```python
from build123d import *

# Parameters (mm, degrees)
SKETCH1_R               = 17
BOSS_EXTRUDE1_DEPTH     = 4.4
CAVITY1_OUTLINE_R       = 3.15
CAVITY1_DEPTH           = 3.283595969
CAVITY1_START           = 1.183595969
CAVITY1_2_OUTLINE_R     = 3.15
CAVITY1_2_OUTLINE_R_2   = 1.575
CAVITY1_2_DEPTH         = 2.1
SKETCH9_R               = 12.8
BOSS_EXTRUDE3_DEPTH     = 5.6
BOSS_EXTRUDE8_DEPTH     = 8
SKETCH2_R               = 0.6
CUT_EXTRUDE1_DEPTH      = 31.033314835
CIRPATTERN1_COUNT       = 6
CUT_EXTRUDE3_DEPTH      = 31.033314835
CUT_EXTRUDE3_DEPTH_BACK = 4
SKETCH4_R               = 4
SKETCH6_R               = 1.8
CUT_EXTRUDE4_DEPTH      = 31.033314835
FILLET1_START           = 10
FILLET1_DEPTH           = 9
CUT_EXTRUDE5_DEPTH      = 27.038433133
CUT_EXTRUDE5_DEPTH_BACK = 5.6


with BuildPart() as part:
    # Sketch1 → Boss-Extrude1 (new body)
    with BuildSketch(Plane.XY):
        Circle(SKETCH1_R)
    extrude(amount=BOSS_EXTRUDE1_DEPTH)

    # Cavity1: read off the stored shape, not the designer's step
    # Cavity1 outline → Cavity1 (cut)
    with BuildSketch(Plane.XY):
        with BuildLine():
            Line((3.9375, 6.819950055), (2.048148228, 15.163776711))
            ThreePointArc((2.048148228, 15.163776711), (0, 16.8), (-2.048148228, 15.163776711))
            Line((-2.048148228, 15.163776711), (-3.9375, 6.819950055))
            Line((-3.9375, 6.819950055), (-12.108141735, 9.355636751))
            ThreePointArc((-12.108141735, 9.355636751), (-14.549226784, 8.4), (-14.156289963, 5.80813996))
            Line((-14.156289963, 5.80813996), (-7.875, 0))
            Line((-7.875, 0), (-14.156289963, -5.80813996))
            ThreePointArc((-14.156289963, -5.80813996), (-14.549226784, -8.4), (-12.108141735, -9.355636751))
            Line((-12.108141735, -9.355636751), (-3.9375, -6.819950055))
            Line((-3.9375, -6.819950055), (-2.048148228, -15.163776711))
            ThreePointArc((-2.048148228, -15.163776711), (0, -16.8), (2.048148228, -15.163776711))
            Line((2.048148228, -15.163776711), (3.9375, -6.819950055))
            Line((3.9375, -6.819950055), (12.108141735, -9.355636751))
            ThreePointArc((12.108141735, -9.355636751), (14.549226784, -8.4), (14.156289963, -5.80813996))
            Line((14.156289963, -5.80813996), (7.875, 0))
            Line((7.875, 0), (14.156289963, 5.80813996))
            ThreePointArc((14.156289963, 5.80813996), (14.549226784, 8.4), (12.108141735, 9.355636751))
            Line((12.108141735, 9.355636751), (3.9375, 6.819950055))
        make_face()
        Circle(CAVITY1_OUTLINE_R, mode=Mode.SUBTRACT)
    extrude(amount=CAVITY1_DEPTH, mode=Mode.SUBTRACT)

    # Cavity1 2 outline → Cavity1 2 (cut)
    with BuildSketch(Plane.XY.offset(CAVITY1_START)):
        Circle(CAVITY1_2_OUTLINE_R)
        Circle(CAVITY1_2_OUTLINE_R_2, mode=Mode.SUBTRACT)
    extrude(amount=CAVITY1_2_DEPTH, mode=Mode.SUBTRACT)

    # Sketch9 → Boss-Extrude3 (add)
    with BuildSketch(Plane.XY.offset(4.4)):
        Circle(SKETCH9_R)
    extrude(amount=BOSS_EXTRUDE3_DEPTH)

    # Sketch12 → Boss-Extrude8 (add)
    with BuildSketch(Plane.XY.offset(10)):
        Polygon((3.9, -6.75499815), (7.8, 0), (3.9, 6.75499815), (-3.9, 6.75499815), (-7.8, 0), (-3.9, -6.75499815), align=None)
    extrude(amount=BOSS_EXTRUDE8_DEPTH)

    # Sketch2 → Cut-Extrude1 (cut, through all)
    with BuildSketch(Plane(origin=(0, 0, 0), x_dir=(-1, 0, 0), z_dir=(0, 0, -1))):
        with Locations(Location((0, 13.5, 0), (0, 0, 180))):
            Circle(SKETCH2_R)
        with Locations(Location((0, 10.5, 0), (0, 0, 180))):
            Circle(SKETCH2_R)
        with Locations(Location((0, 7.5, 0), (0, 0, 180))):
            Circle(SKETCH2_R)
    cut_extrude1 = extrude(amount=-CUT_EXTRUDE1_DEPTH, mode=Mode.SUBTRACT)

    # CirPattern1: Cut-Extrude1 ×6 about axis
    cirpattern1_axis = Axis((0, 0, 0), (0, 0, 1))
    for i in range(1, CIRPATTERN1_COUNT):
        add(cut_extrude1.rotate(cirpattern1_axis, i * 360 / CIRPATTERN1_COUNT), mode=Mode.SUBTRACT)

    # Sketch4 → Cut-Extrude3 (cut, two sides: drawn at the far end of the back side and taken through both)
    with BuildSketch(Plane.XY.offset(-CUT_EXTRUDE3_DEPTH_BACK)):
        Circle(SKETCH4_R)
    extrude(amount=CUT_EXTRUDE3_DEPTH + CUT_EXTRUDE3_DEPTH_BACK, mode=Mode.SUBTRACT)

    # Sketch6 → Cut-Extrude4 (cut, through all)
    with BuildSketch(Plane(origin=(0, 0, 0), x_dir=(-1, 0, 0), z_dir=(0, 0, -1))):
        with Locations(Location((-7.875, 0, 0), (0, 0, 302.067932294))):
            Circle(SKETCH6_R)
        with Locations(Location((7.875, 0, 0), (0, 0, 42.758730598))):
            Circle(SKETCH6_R)
    extrude(amount=-CUT_EXTRUDE4_DEPTH, mode=Mode.SUBTRACT)

    # Fillet1: read off the stored shape, not the designer's step
    # Fillet1 outline → Fillet1 (cut)
    with BuildSketch(Plane.XY.offset(FILLET1_START)):
        with BuildLine():
            Line((-3.9, 6.75499815), (-6.786751346, 1.75499815))
            add(Edge.make_bspline(
                [(-6.786751346, 1.75499815), (-3.9, 6.75499815), (1.873502692, 6.75499815)],
                knots=[0, 0, 0, 1, 1, 1], degree=2, weights=[1, 9, 1]))
            Line((1.873502692, 6.75499815), (-3.9, 6.75499815))
        make_face()
    extrude(amount=FILLET1_DEPTH, mode=Mode.SUBTRACT)

    # Sketch12<4> → Cut-Extrude5 (cut, two sides: drawn at the far end of the back side and taken through both)
    with BuildSketch(Plane.XY.offset(10).offset(-CUT_EXTRUDE5_DEPTH_BACK)):
        Polygon((3.9, -6.75499815), (7.8, 0), (3.9, 6.75499815), (-3.9, 6.75499815), (-7.8, 0), (-3.9, -6.75499815), align=None)
    extrude(amount=CUT_EXTRUDE5_DEPTH + CUT_EXTRUDE5_DEPTH_BACK, mode=Mode.SUBTRACT)


solid = part.part
```
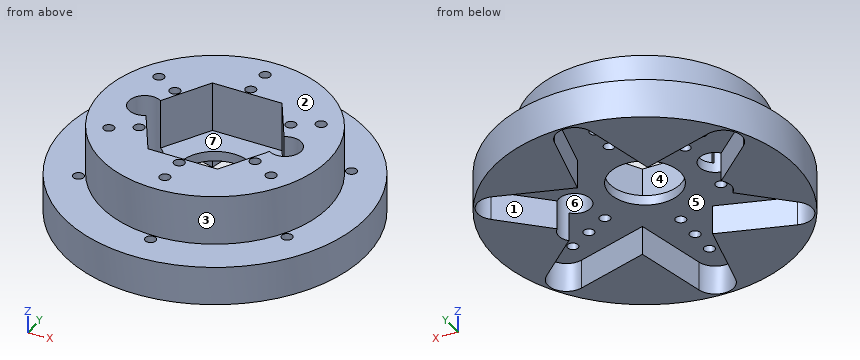
Read the model definition and answer for the solid it produces. Units are mm, in the model's axes. Face numbers are marked on the shaded views. A direction names the side the tool comes from. Give positions to 0.01 mm unless a question says otherwise; leave off trailing zeros. Loops run counter-clockwise (first coordinate to the right, second up) from the corner with the lowest first, then second, coordinate; pieces in that order, holes last.
Item 1: The part is cut by section B-B (z = 6). Give the number of separate pieces and of enclosed holes in the cut face, and give its area (3 significant figures).
Item 2: For the marked faces 5, 6 and 7, determine the directions among +Z, -Z, +X, -X, +Y, -Y from which every point of the face is accessible in a straight line to the end or side of a thin tool.
Item 3: Find the intervals of material crossed by line 1 along Y through (x, z) = (14, 2); line 2 along X through (y, z) = (-5, 5.75); line 3 along Y through (x, z) = (7, 5), in increasing order.
Item 4: The part is cut by section A-A (y = 13.5). Write down the section's boundary in (x, z), and give its area (3 significant figures).
Item 5: The part is cut by section C-C (y = -5.25). Write down the section's boundary in (x, z).
Item 6: Each of these flat-tipped pins is pushed along its axis until it touches: pin 1 Ø9 at (x, y) = (0, 0) entering from -Z; pin 2 Ø5 at (x, y) = (3, 2.5) entering from +Z; pin 3 Ø6 at (x, z) = (13.5, 7) entering from -Y. Where does it stop, or does it pass through?
Item 7: The mould has two halves that part along Y. Classify the marked faces 1, 2, 3 and 4: released by +Y, released by -Y, zero draft, split by the parting line, or undercut.
Taken from the geometry:
1. separate pieces: 1
1. enclosed holes: 13
1. area: 329 mm2
2. face 5: -Z
2. face 6: +Z, -Z
2. face 7: +Z
3. line 1: y = -9.64 to -9.02, -5.66 to 5.66, 9.02 to 9.64
3. line 2: x = -11.78 to -9.64, -8.55 to -4.91, 4.91 to 8.55, 9.64 to 11.78
3. line 3: y = -10.72 to -4.07, -3.43 to -1.57, 1.57 to 3.43, 4.07 to 10.72
4. outline: (-10.33, 0) - (-2.42, 0) - (-2.42, 3.28) - (-0.6, 3.28) - (-0.6, 4.4) - (-10.33, 4.4) - close; (0.6, 3.28) - (2.42, 3.28) - (2.42, 0) - (10.33, 0) - (10.33, 4.4) - (0.6, 4.4) - close
4. area: 73.7 mm2
5. outline: (-16.17, 0) - (-13.55, 0) - (-13.55, 3.28) - (-9.69, 3.28) - (-9.69, 10) - (-11.67, 10) - (-11.67, 4.4) - (-16.17, 4.4) - close; (-8.49, 3.28) - (8.49, 3.28) - (8.49, 10) - (4.77, 10) - (4.77, 4.4) - (-4.77, 4.4) - (-4.77, 10) - (-8.49, 10) - close; (9.69, 3.28) - (13.55, 3.28) - (13.55, 0) - (16.17, 0) - (16.17, 4.4) - (11.67, 4.4) - (11.67, 10) - (9.69, 10) - close
6. pin 1: stops at z = 3.28
6. pin 2: stops at z = 4.4
6. pin 3: stops at y = -12.04
7. face 1: undercut
7. face 2: zero draft
7. face 3: split by the parting line
7. face 4: undercut
